Verification items for the finished model (mm, model axes). Face numbers are marked on the shaded views. A direction names the side the tool comes from. Coordinates: 2 decimals unless noted, no trailing zeros. Loops run counter-clockwise (first coordinate to the right, second up) from the corner with the lowest first, then second, coordinate; pieces in that order, holes last. Notation, with made-up numbers: (-9.75, -30.75) -> (36.25, -30.75) arc R20 cw to (36.25, -25.75) -> close; hole circle Ø4 at (50, 1). An arc over 180 degrees is marked (long way). Write item = value, one per line.
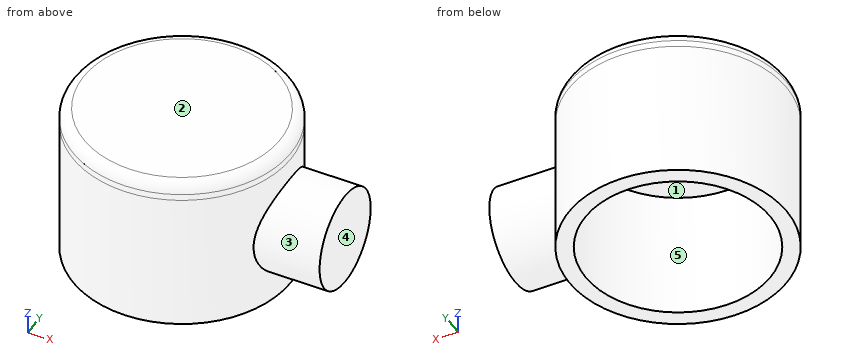
```python
from build123d import *

# Parameters (mm, degrees)
SKETCH2_R             = 50
BOSS_EXTRUDE1_DEPTH   = 64.75
SKETCH4_R             = 50
BOSS_EXTRUDE2_DEPTH   = 8
FILLET1_R             = 5
BODY_MOVE_COPY2_ANGLE = 120
SKETCH5_R             = 42.5
CUT_EXTRUDE1_DEPTH    = 60


with BuildPart() as part:
    # Sketch2 → Boss-Extrude1 (new body)
    with BuildSketch(Plane(origin=(0, 0, 0), x_dir=(0, 0, -1), z_dir=(1, 0, 0))):
        Circle(SKETCH2_R)
    extrude(amount=BOSS_EXTRUDE1_DEPTH)

    # Sketch3 → Revolve1 (revolve)
    with BuildSketch(Plane.ZY.offset(-32.375)):
        with BuildLine():
            Line((0, 75), (0, 50))
            ThreePointArc((0, 50), (11.563490229, 48.644482665), (22.5, 44.651427749))
            Line((22.5, 44.651427749), (22.5, 75))
            Line((22.5, 75), (0, 75))
        make_face()
    revolve(axis=Axis((32.375, 50, 0), (0, 1, 0)))

    # Sketch4 → Boss-Extrude2 (add)
    with BuildSketch(Plane.ZY):
        Circle(SKETCH4_R)
    extrude(amount=BOSS_EXTRUDE2_DEPTH)

    # Fillet1
    fillet1_edges = [part.edges().sort_by_distance(p)[0] for p in [
        (-8, 0, -50),
    ]]
    fillet(fillet1_edges, radius=FILLET1_R)


with BuildPart() as part_1:
    # Body-Move_Copy1: moved
    add(part.part.moved(Location((-32.38, 0, 0))))


with BuildPart() as part_2:
    # Body-Move_Copy2: moved
    add(part_1.part.rotate(Axis((0, 0, 0), (0.577350269, 0.577350269, -0.577350269)), BODY_MOVE_COPY2_ANGLE))

    # Sketch5 → Cut-Extrude1 (cut)
    with BuildSketch(Plane(origin=(0, 0, -32.37), x_dir=(-1, 0, 0), z_dir=(0, 0, -1))):
        Circle(SKETCH5_R)
    extrude(amount=-CUT_EXTRUDE1_DEPTH, mode=Mode.SUBTRACT)


solid = part_2.part
```
1) Release check for a two-part mould opening along Y. For the marked faces 1, 2 and 3 record: pulls with the +Y half, pulls with the -Y half, needs draft (parallel to the pull), parting line crosses it, or undercut.
Ans:
face_1 = undercut
face_2 = needs draft
face_3 = parting line crosses it
2) Depth check by flat-ended pin: pin 1 Ø4 at (x, z) = (50, 16.5) entering from -Y; pin 2 Ø1.5 at (y, z) = (-8.5, 22) entering from +X; pin 3 Ø1.5 at (x, y) = (-23, 27.5) entering from -Z. Enter the tip coordinate at first touch or a pass-through.
Ans:
pin_1 = -17.21
pin_2 = 49.4
pin_3 = 27.63
3) Sectioned sample at C-C, the plane z = -12. Record the cut outline in (x, y).
Ans:
outline = (46.24, -19.03) -> (75, -19.03) -> (75, 19.03) -> (46.24, 19.03) arc R50 ccw (long way) to start; hole circle Ø85 at (0, 0)
4) Sectioned sample at D-D, the plane z = 14. Record the cut outline in (x, y), plus the area to 3 significant figures.
Ans:
outline = (46.79, -17.62) -> (75, -17.62) -> (75, 17.62) -> (46.79, 17.62) arc R50 ccw (long way) to start; hole circle Ø85 at (0, 0)
area = 3,100 mm2
5) Sectioned sample at B-B, the plane x = 0. Record the cut outline in (y, z).
Ans:
outline = (-50, -32.37) -> (-42.5, -32.37) -> (-42.5, 27.63) -> (42.5, 27.63) -> (42.5, -32.37) -> (50, -32.37) -> (50, 35.38) arc R5 ccw to (45, 40.38) -> (-45, 40.38) arc R5 ccw to (-50, 35.38) -> close
6) Sectioned sample at A-A, the plane y = 0. Record the cut outline in (x, z) (3 decimals).
Ans:
outline = (-50, -32.37) -> (-42.5, -32.37) -> (-42.5, 27.63) -> (42.5, 27.63) -> (42.5, -32.37) -> (50, -32.37) -> (50, -22.495) -> (75, -22.495) -> (75, 22.505) -> (50, 22.505) -> (50, 35.38) arc R5 ccw to (45, 40.38) -> (-45, 40.38) arc R5 ccw to (-50, 35.38) -> close
7) Material ranges on line 1 (Y direction, x = 0, z = 8); line 2 (Y direction, x = 17, z = 10.5); line 3 (X direction, y = 27.5, z = -8.5), recorded low to high.
Ans:
line_1 = -50 to -42.5, 42.5 to 50
line_2 = -47.02 to -38.95, 38.95 to 47.02
line_3 = -41.76 to -32.4, 32.4 to 41.76
8) Tool access check on the marked faces 4 and 5. Record the directions out of +Z, -Z, +X, -X, +Y, -Y that give a thin tool (end or side, any length) a straight path to the whole face; none if there is none.
Ans:
face_4 = +Z, -Z, +X, +Y, -Y
face_5 = -Z
